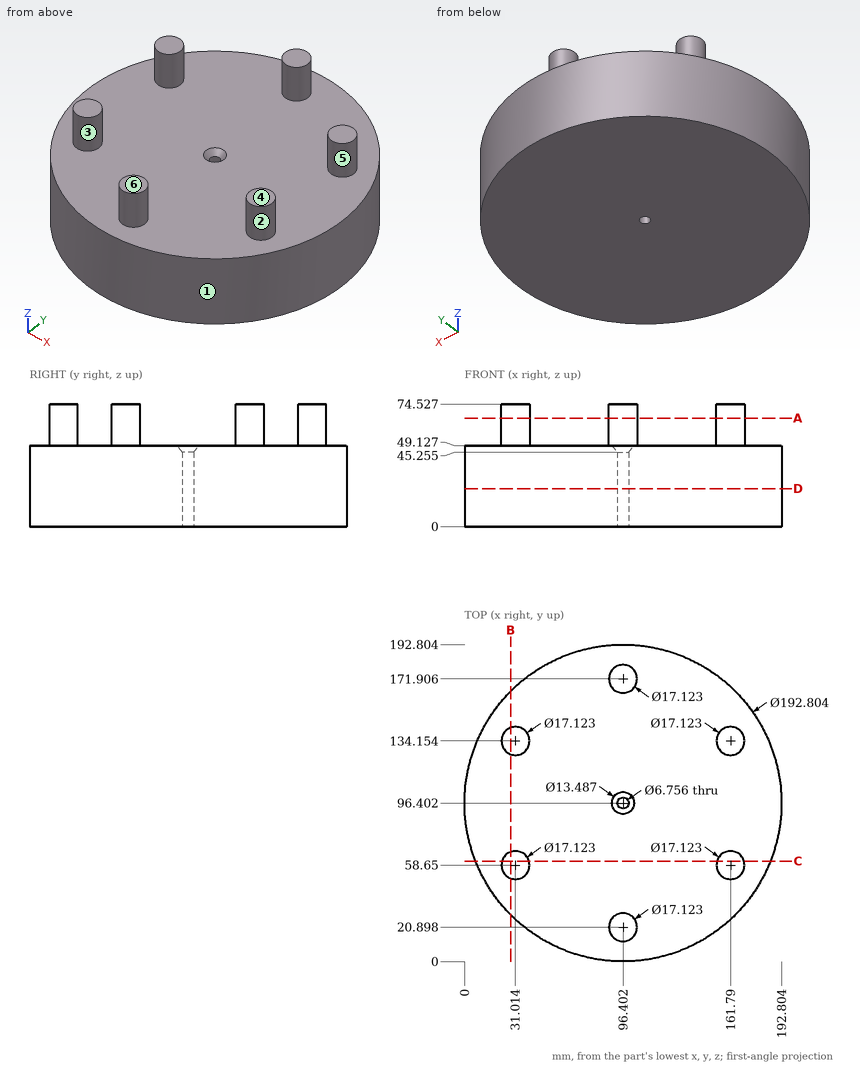
Design review of the part shown in the three views and the two pictorial views. Dimensions are in mm from the part's minimum x, y and z. A direction names the side the tool comes from. Give positions to 0.01 mm unless a question says otherwise; leave off trailing zeros. Write each loop counter-clockwise with the first axis right and the second up, starting at its lowest first coordinate (ties: lowest second). Pieces come first, ordered by that corner, then holes. Notation, with made-up numbers: M 61,-13 L 79,-13 A12 ccw 79,4 Z; hole C -19,0.5 d6. An arc over 180 degrees is marked long. Answer in a Markdown table with one row per item.
Item 1: Add section A-A on z = 66. State how many separate pieces and enclosed holes the cut face has, plus the area to 3 significant figures.
Check sheet entries:
| item | result |
|---|---|
| separate pieces | 6 |
| enclosed holes | 0 |
| area | 1,380 mm2 |
Item 2: For P1, Ø10, axis at x = 155.5, z = 65, coming from the -Y side; P2, Ø4, axis at y = 156.5, z = 8.5, coming from the +X side; P3, Ø5, axis at y = 54, z = 61, coming from the -X side, all flat-tipped, find the tip position at first contact; note any pin that passes through.
Check sheet entries:
| item | result |
|---|---|
| P1 | y = 50.19 |
| P2 | x = 173.33 |
| P3 | x = 22.73 |
Item 3: Add section D-D on z = 23. Give the boundary of the cut face in (x, y).
Check sheet entries:
| item | result |
|---|---|
| outline | C 96.4,96.4 d192.8; hole C 96.4,96.4 d6.76 |
Item 4: Add section B-B on x = 28. Give the boundary of the cut face in (y, z), plus the area to 3 significant figures.
Check sheet entries:
| item | result |
|---|---|
| outline | M 28.47,0 L 164.33,0 L 164.33,49.13 L 142.17,49.13 L 142.17,74.53 L 126.14,74.53 L 126.14,49.13 L 66.66,49.13 L 66.66,74.53 L 50.64,74.53 L 50.64,49.13 L 28.47,49.13 Z |
| area | 7,490 mm2 |
Item 5: Tool access review of the marked faces 5 and 6: name each direction out of +Z, -Z, +X, -X, +Y, -Y from which nothing blocks a thin tool from reaching the whole face with its end or side.
Check sheet entries:
| item | result |
|---|---|
| face 5 | +Z |
| face 6 | +Z, +X, -X, +Y, -Y |
Item 6: Draft analysis for pull direction Y (two halves, no side actions). For the marked faces 1, 2, 3 and 4, state which applies: +Y half, -Y half, draft (parallel to the pull), parting line (faces both ways), or undercut.
Check sheet entries:
| item | result |
|---|---|
| face 1 | parting line |
| face 2 | undercut |
| face 3 | undercut |
| face 4 | draft |
Item 7: Add section C-C on y = 61. Give the boundary of the cut face in (x, z) (1 decimal), plus the area to 3 significant figures.
Check sheet entries:
| item | result |
|---|---|
| outline | M 6.7,0 L 186.1,0 L 186.1,49.1 L 170,49.1 L 170,74.5 L 153.6,74.5 L 153.6,49.1 L 39.2,49.1 L 39.2,74.5 L 22.8,74.5 L 22.8,49.1 L 6.7,49.1 Z |
| area | 9,650 mm2 |
Item 8: For line 1 along Z through (x, y) = (117, 167.5); line 2 along X through (y, z) = (173.5, 40) (1 decimal); line 3 along X through (y, z) = (137.5, 23) (1 decimal), list the stretches that pass through material, from the lowest coordinate up.
Check sheet entries:
| item | result |
|---|---|
| line 1 | 0 to 49.13 |
| line 2 | 38.5 to 154.3 |
| line 3 | 9.2 to 183.6 |
